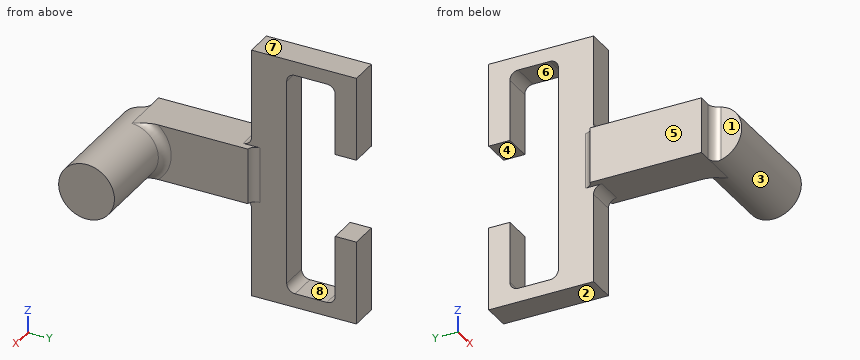
from build123d import *

# Parameters (mm, degrees)
SKETCH2_R           = 12.7
BOSS_EXTRUDE1_DEPTH = 50.8
SKETCH3_W           = 25.4
SKETCH3_H           = 50.8
BOSS_EXTRUDE2_DEPTH = 9.525
SKETCH5_W           = 101.6
SKETCH5_H           = 16.002
BOSS_EXTRUDE3_DEPTH = 6.35
SKETCH6_W           = 6.35
SKETCH6_H           = 38.1
BOSS_EXTRUDE4_DEPTH = 6.35
SKETCH7_W           = 38.1
SKETCH7_H           = 9.652
BOSS_EXTRUDE5_DEPTH = 6.35
FILLET1_R           = 3.81
FILLET2_R           = 3.81


with BuildPart() as part:
    # Sketch2 → Boss-Extrude1 (new body)
    with BuildSketch(Plane(origin=(0, 0, 0), x_dir=(0, 0, -1), z_dir=(1, 0, 0))):
        Circle(SKETCH2_R)
    extrude(amount=BOSS_EXTRUDE1_DEPTH)

    # Sketch3 → Boss-Extrude2 (add, symmetric)
    with BuildSketch(Plane.ZY):
        with Locations((0.014597196, 26.008732875)):
            Rectangle(SKETCH3_W, SKETCH3_H)
    extrude(amount=BOSS_EXTRUDE2_DEPTH, both=True)


with BuildPart() as body_2:
    # Sketch5 → Boss-Extrude3 (new, symmetric)
    with BuildSketch(Plane(origin=(0, 0, 0), x_dir=(0, 0, -1), z_dir=(1, 0, 0))):
        with Locations((0, 59.392294155)):
            Rectangle(SKETCH5_W, SKETCH5_H)
    extrude(amount=BOSS_EXTRUDE3_DEPTH, both=True)

    # Sketch6 → Boss-Extrude4 (add, symmetric)
    with BuildSketch(Plane(origin=(0, 0, 0), x_dir=(0, 0, -1), z_dir=(1, 0, 0))):
        with Locations((-53.975, 70.441294155)):
            Rectangle(SKETCH6_W, SKETCH6_H)
        with Locations((53.975, 70.441294155)):
            Rectangle(SKETCH6_W, SKETCH6_H)
    extrude(amount=BOSS_EXTRUDE4_DEPTH, both=True)

    # Sketch7 → Boss-Extrude5 (add, symmetric)
    with BuildSketch(Plane(origin=(0, 0, 0), x_dir=(0, 0, -1), z_dir=(1, 0, 0))):
        with Locations((-38.1, 94.317294155)):
            Rectangle(SKETCH7_W, SKETCH7_H)
        with Locations((38.1, 94.317294155)):
            Rectangle(SKETCH7_W, SKETCH7_H)
    extrude(amount=BOSS_EXTRUDE5_DEPTH, both=True)


with BuildPart() as part_1:
    add(part.part)

    # Combine1: union body 2
    add(body_2.part)

    # Fillet1
    # the kernel refuses this fillet: 3.81 mm, written as the material it adds along each edge
    with BuildSketch(Plane(origin=(-6.35, 51.391294155, 12.714597196), x_dir=(0, -1, 0), z_dir=(1, 0, 0)), Plane(origin=(6.35, 51.391294155, -12.685402804), x_dir=(0, -1, 0), z_dir=(-1, 0, 0)), Plane(origin=(6.35, 67.393294155, -50.8), x_dir=(0, 1, 0), z_dir=(-1, 0, 0)), Plane(origin=(-6.35, 89.491294155, 50.8), x_dir=(0, 0, -1), z_dir=(1, 0, 0)), Plane(origin=(-6.35, 67.393294155, 50.8), x_dir=(0, 1, 0), z_dir=(1, 0, 0))) as fillet1_piece_1:
        with BuildLine():
            CenterArc((FILLET1_R, -FILLET1_R), FILLET1_R, 90, 90)
            Line((0, -FILLET1_R), (0, 0))
            Line((0, 0), (FILLET1_R, 0))
        make_face()
    extrude(amount=12.7)
    with BuildSketch(Plane(origin=(9.525, 0, 0), x_dir=(0, -0.6466492608489325, 0.762787475935158), z_dir=(0, -0.762787475935158, -0.6466492608489325))) as fillet1_piece_2_section:
        with BuildLine():
            CenterArc((12.7 + FILLET1_R, -FILLET1_R), FILLET1_R, 90, 90)
            Line((12.7 + FILLET1_R, 0), (12.7, 0))
            Line((12.7, 0), (12.7, -FILLET1_R))
        make_face()
    fillet1_piece_2 = revolve(axis=Axis((9.525, 0, 0), (-1, 0, 0)), revolution_arc=260.578888602, mode=Mode.PRIVATE)
    fillet1_piece_2 = split(fillet1_piece_2, bisect_by=Plane(origin=(10.607555303, 13.782555283, -12.685402804), z_dir=(0, 0, 1)), keep=Keep.TOP, mode=Mode.PRIVATE)
    fillet1_piece_2 = split(fillet1_piece_2, bisect_by=Plane(origin=(10.607555303, 0.608732875, 0.000757571), z_dir=(0, 1, 0)), keep=Keep.TOP, mode=Mode.PRIVATE)
    fillet1_piece_2 = split(fillet1_piece_2, bisect_by=Plane(origin=(10.607555303, 13.782555283, 12.714597196), z_dir=(0, 0, -1)), keep=Keep.TOP, mode=Mode.PRIVATE)
    add(fillet1_piece_2)
    with BuildSketch(Plane(origin=(6.35, 89.491294155, -50.8), x_dir=(0, -1, 0), z_dir=(-1, 0, 0))) as fillet1_piece_3:
        with BuildLine():
            CenterArc((FILLET1_R, FILLET1_R), FILLET1_R, 180, 90)
            Line((0, FILLET1_R), (0, 0))
            Line((0, 0), (FILLET1_R, 0))
        make_face()
    extrude(amount=12.7)

    # Fillet2
    # the kernel refuses this fillet: 3.81 mm, written as the material it adds along each edge
    with BuildSketch(Plane(origin=(0, 0.608732875, 22.210402804), x_dir=(-1, 0, 0), z_dir=(0, 0, -1))) as fillet2_piece_1_section:
        with BuildLine():
            CenterArc((FILLET2_R, -FILLET2_R), FILLET2_R, 90, 90)
            Line((0, -FILLET2_R), (0, 0))
            Line((0, 0), (FILLET2_R, 0))
        make_face()
    fillet2_piece_1 = extrude(amount=44.420805607, mode=Mode.PRIVATE)
    fillet2_piece_1 = fillet2_piece_1 & Plane(origin=(-0.851863451, 0, 0), x_dir=(0, 0, -1), z_dir=(-1, 0, 0)) * Cylinder(12.7, 105, mode=Mode.PRIVATE)
    add(fillet2_piece_1)
    with BuildSketch(Plane(origin=(-6.35, 51.408732875, 12.714597196), x_dir=(0, 1, 0), z_dir=(0, 0, -1))) as fillet2_piece_2:
        with BuildLine():
            CenterArc((3.756710662, -3.81), FILLET2_R, 90, 80.405931773)
            Line((0, -3.175), (0, 0))
            Line((0, 0), (3.756710662, 0))
        make_face()
    extrude(amount=25.4)
    with BuildSketch(Plane(origin=(6.35, 51.408732875, 12.714597196), x_dir=(0, 1, 0), z_dir=(0, 0, -1))) as fillet2_piece_3:
        with BuildLine():
            CenterArc((3.756710662, 3.81), FILLET2_R, 189.594068227, 80.405931773)
            Line((0, 3.175), (0, 0))
            Line((0, 0), (3.756710662, 0))
        make_face()
    extrude(amount=25.4)


solid = part_1.part
Could you check a few things on this model? Use its own coordinates, in mm. Face numbers are marked on the shaded views. A direction names the side the tool comes from. Give positions to 0.01 mm unless a question says otherwise; leave off trailing zeros. Loops run counter-clockwise (first coordinate to the right, second up) from the corner with the lowest first, then second, coordinate; pieces in that order, holes last. Notation, with made-up numbers: (18, -13) -> (42, -13) arc R13 cw to (42, 5) -> close; hole circle Ø1 at (-21, -20). An arc over 180 degrees is marked (long way). Return JSON: item names as keys, results as strings.
Item 1: I'm going to push flat-ended pins straight in: pin 1 (14 mm diameter, centred on x = 0, z = -5, fed in from +Y); pin 2 (25 mm diameter, centred on x = 3, y = 33.5, fed in from -Z); pin 3 (24.5 mm diameter, centred on x = 4.5, y = 23, fed in from +Z). Where does each tip first touch, or does it pass through?
Geometry results:
{"pin 1": "stops at y = 67.39", "pin 2": "stops at z = -12.69", "pin 3": "stops at z = 12.71"}
Item 2: If we section it at C-C on z = 0: List the corners of the cut face in (x, y) for me (3 decimals).
Geometry results:
{"outline": "(-9.525, 0.609) -> (-3.81, 0.609) arc R3.81 cw to (0, -3.201) -> (0, -12.7) -> (50.8, -12.7) -> (50.8, 12.7) -> (13.335, 12.7) arc R3.81 cw to (9.525, 16.51) -> (9.525, 51.409) arc R3.81 cw to (6.35, 55.165) -> (6.35, 67.393) -> (-6.35, 67.393) -> (-6.35, 55.165) arc R3.81 cw to (-9.525, 51.409) -> close"}
Item 3: I need wall thicknesses on L1, parallel to Y at x = 1, z = -27.5; L2, parallel to X at y = -3, z = -8; L3, parallel to X at y = 52.5, z = -27.5. Which ranges of each line are inside material? Lowest first, please. Write a range as from..to.
Geometry results:
{"L1": "y = 51.39..67.39, 89.49..99.14", "L2": "x = -0.01..50.8", "L3": "x = -6.35..6.35"}
Item 4: If we section it at A-A on y = 92: List the corners of the cut face in (x, z) for me, plus the area to 3 significant figures.
Geometry results:
{"outline": "(-6.35, -57.15) -> (6.35, -57.15) -> (6.35, -19.05) -> (-6.35, -19.05) -> close; (-6.35, 19.05) -> (6.35, 19.05) -> (6.35, 57.15) -> (-6.35, 57.15) -> close", "area": "968 mm²"}
Item 5: We'd pull the mould along Y, two halves only. Please class the marked faces 6, 7 and 8: +Y half, -Y half, draft (parallel to the pull), parting line (faces both ways), or undercut.
Geometry results:
{"face 6": "undercut", "face 7": "draft", "face 8": "undercut"}
Item 6: If we section it at B-B on z = 33.5: List the corners of the cut face in (x, y) for me.
Geometry results:
{"outline": "(-6.35, 51.39) -> (6.35, 51.39) -> (6.35, 67.39) -> (-6.35, 67.39) -> close; (-6.35, 89.49) -> (6.35, 89.49) -> (6.35, 99.14) -> (-6.35, 99.14) -> close"}
Item 7: Which directions (+Z, -Z, +X, -X, +Y, -Y) give clear straight access to the entire face, cutting with the end or side of a thin tool? Please do the marked faces 1, 2, 3, 4 and 5.
Geometry results:
{"face 1": "+Z, -Z, -X, -Y", "face 2": "-Z, +X, -X, +Y, -Y", "face 3": "+X", "face 4": "+X, -X, +Y", "face 5": "+Z, -Z, -X, +Y, -Y"}
